Autodesk Inventor part; units mm, degrees
ref_plane "YZ Plane" through (0, 0, 0) normal (1, 0, 0) x (0, 1, 0)
ref_plane "XZ Plane" through (0, 0, 0) normal (0, 1, 0) x (-1, 0, 0)
ref_plane "XY Plane" through (0, 0, 0) normal (0, 0, 1) x (1, 0, 0)
sketch "Connector Hole Layout" plane through (0, 0, 0) normal (0, 1, 0) x (-1, 0, 0)
  circle A0 centre (42.948752, 7.963756) radius 1.6 construction
  circle A1 centre (-17.538767, 30.213756) radius 1.6 construction
  circle A2 centre (42.948752, 52.463756) radius 1.6 construction
  line L0 (42.948752, 7.963756) -> (42.948752, 52.463756) construction
  line L1 (41.447122, 51.91139) -> (-16.037138, 30.766122) construction
  point P0 (42.948752, 30.213756)
  dimension "d0" = 3.2
  dimension "d22" = 44.5
  dimension "d23" = 61.25
sketch "Sketch8" plane through (0, 0, 0) normal (0, 1, 0) x (-1, 0, 0)
  circle A0 centre (42.948752, 7.963756) radius 1.6 construction
  circle A1 centre (42.948752, 52.463756) radius 1.6 construction
  circle A2 centre (-17.538767, 30.213756) radius 1.6 construction
  circle A3 centre (42.948752, 7.963756) radius 4
  point P0 (0, 0)
  dimension "d51" = 8
sketch "Sketch8 outline for Extrusion5" plane through (0, 0, 0) normal (0, 1, 0) x (-1, 0, 0)
  circle A0 centre (42.948752, 7.963756) radius 4
extrude "Extrusion5" add sketch "Sketch8 outline for Extrusion5" along normal blind 7
sketch "Sketch9" plane through (-42.948752, 7, 7.963756) normal (0, 1, 0) x (1, 0, 0)
  point P0 (42.948752, 7.963756)
  point P1 (0, 0)
hole "Hole2" at (-42.948752, 7, 7.963756) direction (0, -1, 0) diameter 4 depth 5 tip angle 118
chamfer "Chamfer3" distance 1 distance2 2 1 edges at (-38.9488, 7, 7.9638) measured on face at (-46.2385, 7, 7.5643)
pattern_sketch "Sketch Driven Pattern1" from (-42.948752, 0, 7.963756) copies at (-42.948752, 0, 52.463756) at (17.538767, 0, 30.213756)
sketch "Sketch10" plane through (-42.948752, 0, 52.463756) normal (0, -1, 0) x (1, 0, 0)
  circle A0 centre (0, 0) radius 4
  line L0 (1.380915, 3.754074) -> (61.868435, -18.495926)
  circle A1 centre (60.487519, -22.25) radius 4
  line L1 (61.868435, -26.004074) -> (1.380915, -48.254074)
  circle A2 centre (0, -44.5) radius 4
  line L2 (-4, -44.5) -> (-4, 0)
  circle A3 centre (0, 0) radius 4
  circle A4 centre (0, -44.5) radius 4
  point P0 (42.948752, -52.463756)
sketch "Sketch10 outline for Extrusion6" plane through (-42.948752, 0, 52.463756) normal (0, -1, 0) x (1, 0, 0)
  line L0 (-4, 0) -> (-4, -44.5)
  arc A0 (1.380915, 3.754074) -> (-4, 0) centre (0, 0) ccw
  line L1 (61.868435, -18.495926) -> (1.380915, 3.754074)
  arc A1 (61.868435, -26.004074) -> (61.868435, -18.495926) centre (60.487519, -22.25) ccw
  line L2 (1.380915, -48.254074) -> (61.868435, -26.004074)
  arc A2 (-4, -44.5) -> (1.380915, -48.254074) centre (0, -44.5) ccw
extrude "Extrusion6" add sketch "Sketch10 outline for Extrusion6" along normal blind 4.5
sketch "Sketch11" plane through (-42.948752, 0, 52.463756) normal (0, 1, 0) x (1, 0, 0)
  line L0 (-4, 48.5) -> (64.487519, 48.5) construction
  line L1 (64.487519, 48.5) -> (64.487519, -4) construction
  line L2 (64.487519, -4) -> (-4, -4) construction
  line L3 (-4, -4) -> (-4, 48.5) construction
  circle A0 centre (60.487519, 22.25) radius 4 construction
  circle A1 centre (0, 0) radius 4 construction
  circle A2 centre (0, 44.5) radius 4 construction
  line L4 (30.24376, 48.5) -> (30.24376, -4) construction
  line L5 (-4, 22.25) -> (64.487519, 22.25) construction
  line L6 (16.27376, 22.25) -> (18.81376, 22.25) construction
  line L7 (16.27376, 19.65) -> (18.81376, 19.65)
  line L8 (18.81376, 24.85) -> (16.27376, 24.85)
  arc A3 (16.27376, 24.85) -> (16.27376, 19.65) centre (16.27376, 22.25) ccw
  arc A4 (18.81376, 19.65) -> (18.81376, 24.85) centre (18.81376, 22.25) ccw
  line L9 (44.21376, 19.65) -> (41.67376, 19.65)
  line L10 (41.67376, 24.85) -> (44.21376, 24.85)
  arc A5 (44.21376, 19.65) -> (44.21376, 24.85) centre (44.21376, 22.25) ccw
  arc A6 (41.67376, 24.85) -> (41.67376, 19.65) centre (41.67376, 22.25) ccw
  point P0 (42.948752, 52.463756)
  point P1 (30.24376, 22.25)
  point P2 (30.24376, 22.25)
  point P3 (17.54376, 22.25)
  point P4 (17.54376, 24.85)
  point P5 (17.54376, 19.65)
  dimension "d66" = 11.43
  dimension "d67" = 13.97
  dimension "d68" = 5.2
sketch "Sketch11 outline for Extrusion7" plane through (-42.948752, 0, 52.463756) normal (0, 1, 0) x (1, 0, 0)
  arc A0 (44.21376, 19.65) -> (44.21376, 24.85) centre (44.21376, 22.25) ccw
  line L0 (41.67376, 19.65) -> (44.21376, 19.65)
  arc A1 (41.67376, 24.85) -> (41.67376, 19.65) centre (41.67376, 22.25) ccw
  line L1 (44.21376, 24.85) -> (41.67376, 24.85)
  line L2 (16.27376, 19.65) -> (18.81376, 19.65)
  arc A2 (16.27376, 24.85) -> (16.27376, 19.65) centre (16.27376, 22.25) ccw
  line L3 (18.81376, 24.85) -> (16.27376, 24.85)
  arc A3 (18.81376, 19.65) -> (18.81376, 24.85) centre (18.81376, 22.25) ccw
extrude "Extrusion7" cut sketch "Sketch11 outline for Extrusion7" against normal blind 10
properties part number "db-25_standoffs_plate_t-slot-2inx1in"
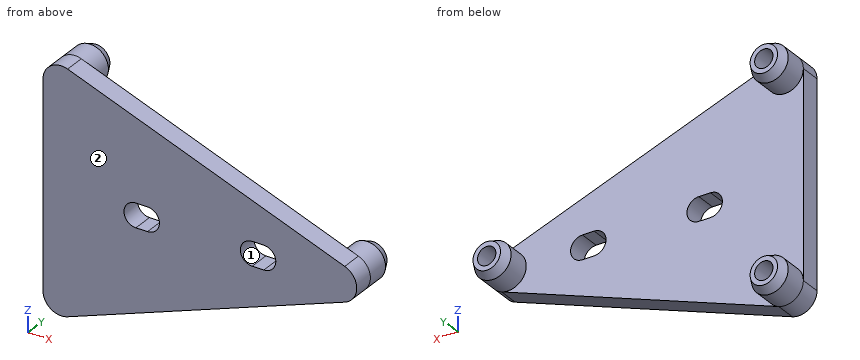
The listing builds one solid part. Answer for the finished solid, in the listing's coordinates (mm). Face numbers are marked on the shaded views. Give positions to 0.01 mm unless a question says otherwise; leave off trailing zeros. Write each loop counter-clockwise with the first axis right and the second up, starting at its lowest first coordinate (ties: lowest second). Pieces come first, ordered by that corner, then holes.
Item 1: Flat-ended cylindrical pins translate along their axes: P1, Ø0.8, axis at x = -26, y = -3, coming from the +Z side; P2, Ø1, axis at x = -10.5, z = 30.5, coming from the +Y side; P3, Ø1.5, axis at x = 3.5, z = 42, coming from the +Y side; P4, Ø3, axis at x = -19.5, y = -0.5, coming from the +Z side. Find the tip coordinate at first contact, or state that the pin passes through.
Item 2: Section A-A, the plane x = -2.5 is taken. Write down the section's boundary in (y, z).
Item 3: Section B-B, the plane y = -2 is taken. Write down the section's boundary in (x, z) (3 decimals).
Item 4: Section C-C, the plane y = 3 is taken. Write down the section's boundary in (x, z), plus the area to 3 significant figures.
Item 5: Section D-D, the plane z = 25 is taken. Write down the section's boundary in (x, y).
Item 6: Determine the mould class of the marked faces 1 and 2 for opening direction Z: released by +Z, released by -Z, zero draft, split by the parting line, or undercut.
Item 7: Find the intervals of material crossed by line 1 along Z through (x, y) = (-42.5, 4); line 2 along Z through (x, y) = (-3, -1.5); line 3 along Y through (x, z) = (-39.5, 19.5), in increasing order.
Completed:
1. P1: stops at z = 50.64
1. P2: stops at y = 0
1. P3: passes through
1. P4: stops at z = 48.65
2. outline: (-4.5, 18.58) - (0, 18.58) - (0, 27.92) - (-4.5, 27.92) - close; (-4.5, 32.51) - (0, 32.51) - (0, 41.85) - (-4.5, 41.85) - close
3. outline: (-46.949, 7.964) arc R4 ccw to (-41.568, 4.21) - (18.92, 26.46) arc R4 ccw to (18.92, 33.968) - (-41.568, 56.218) arc R4 ccw to (-46.949, 52.464) - close; hole (-26.675, 27.614) - (-24.135, 27.614) arc R2.6 ccw to (-24.135, 32.814) - (-26.675, 32.814) arc R2.6 ccw to start; hole (-1.275, 27.614) - (1.265, 27.614) arc R2.6 ccw to (1.265, 32.814) - (-1.275, 32.814) arc R2.6 ccw to start
4. outline: circle Ø8 at (-42.95, 7.96); circle Ø8 at (-42.95, 52.46); circle Ø8 at (17.54, 30.21); hole circle Ø4 at (-42.95, 7.96); hole circle Ø4 at (-42.95, 52.46); hole circle Ø4 at (17.54, 30.21)
4. area: 113 mm2
5. outline: (-46.95, -4.5) - (14.95, -4.5) - (14.95, 0) - (-46.95, 0) - close
6. face 1: undercut
6. face 2: zero draft
7. line 1: z = 3.99 to 6.01, 9.91 to 11.94, 48.49 to 50.51, 54.41 to 56.44
7. line 2: z = 18.4 to 28.27, 32.16 to 42.03
7. line 3: y = -4.5 to 0
